Model file for the job. Use its own axes, mm. Round coordinates to 2 decimals unless told otherwise and drop trailing zeros. Loops run counter-clockwise (first coordinate to the right, second up) from the corner with the lowest first, then second, coordinate; pieces in that order, holes last. Notation, with made-up numbers: M -35.5,-27 L -19.5,-27 A19 ccw -19.5,-3 Z; hole C 62.5,32 d5. An arc over 180 degrees is marked long. Answer in a Markdown table with one row per item.
from build123d import *

# Parameters (mm, degrees)
SKETCH3_W                    = 720
SKETCH3_H                    = 30
BASE_FLANGE1_DEPTH           = 3
EDGE_FLANGE1_STRIP_W         = 13.4732
EDGE_FLANGE1_STRIP_H         = 3
EDGE_FLANGE1_STRIP_CUT_DEPTH = 720
EDGE_FLANGE1_DEPTH           = 720
SKETCH10_R                   = 5
CUT_EXTRUDE2_DEPTH           = 10
SKETCH11_R                   = 5
CUT_EXTRUDE3_DEPTH           = 10
SKETCH12_R                   = 5
CUT_EXTRUDE4_DEPTH           = 10


# Sheet-metal steps are written as plain solids
with BuildPart() as part:
    # Sketch3 → Base-Flange1 (new body)
    with BuildSketch(Plane(origin=(0, 0, 0), x_dir=(1, 0, 0), z_dir=(0, 1, 0))):
        Rectangle(SKETCH3_W, SKETCH3_H)
    extrude(amount=-BASE_FLANGE1_DEPTH)

    # Edge-Flange1 strip (across the edge) → Edge-Flange1 strip cut (cut)
    with BuildSketch(Plane(origin=(360, 0, -15), x_dir=(0, 0, 1), z_dir=(-1, 0, 0))):
        with Locations((-6, -1.5)):
            Rectangle(EDGE_FLANGE1_STRIP_W, EDGE_FLANGE1_STRIP_H)
    extrude(amount=EDGE_FLANGE1_STRIP_CUT_DEPTH, mode=Mode.SUBTRACT)

    # Edge-Flange1 section (across the edge) → Edge-Flange1 (add)
    with BuildSketch(Plane(origin=(360, 0, -15), x_dir=(0, 0, 1), z_dir=(-1, 0, 0))):
        with BuildLine():
            Line((-3, 0.7366), (-3, 27))
            Line((-3, 27), (0, 27))
            Line((0, 27), (0, 0.7366))
            ThreePointArc((0, 0.7366), (0.215745145, 0.215745145), (0.7366, 0))
            Line((0.7366, 0), (0.7366, -3))
            ThreePointArc((0.7366, -3), (-1.905575199, -1.905575199), (-3, 0.7366))
        make_face()
    extrude(amount=EDGE_FLANGE1_DEPTH)

    # Sketch10 → Cut-Extrude2 (cut)
    with BuildSketch(Plane(origin=(0, 0, 0), x_dir=(1, 0, 0), z_dir=(0, 1, 0))):
        with Locations(Location((-340, -1, 0), (0, 0, 270))):
            Circle(SKETCH10_R)
        with Locations(Location((-320, -1, 0), (0, 0, 270))):
            Circle(SKETCH10_R)
    cut_extrude2 = extrude(amount=-CUT_EXTRUDE2_DEPTH, mode=Mode.SUBTRACT)

    # Mirror1: Cut-Extrude2 across plane
    add(cut_extrude2.mirror(Plane(origin=(0, 0, 0), x_dir=(0, 0, 1), z_dir=(1, 0, 0))), mode=Mode.SUBTRACT)

    # Sketch11 → Cut-Extrude3 (cut)
    with BuildSketch(Plane.XY.offset(-15)):
        with Locations((225.5, 17)):
            Circle(SKETCH11_R)
        with Locations((-225.5, 17)):
            Circle(SKETCH11_R)
        with Locations((-150.5, 17)):
            Circle(SKETCH11_R)
        with Locations((150.5, 17)):
            Circle(SKETCH11_R)
        with Locations((50, 17)):
            Circle(SKETCH11_R)
        with Locations((-50, 17)):
            Circle(SKETCH11_R)
    extrude(amount=-CUT_EXTRUDE3_DEPTH, mode=Mode.SUBTRACT)

    # Sketch12 → Cut-Extrude4 (cut)
    with BuildSketch(Plane(origin=(0, 0, 0), x_dir=(1, 0, 0), z_dir=(0, 1, 0))):
        with Locations(Location((-75, -1, 0), (0, 0, 270))):
            Circle(SKETCH12_R)
        with Locations(Location((75, -1, 0), (0, 0, 270))):
            Circle(SKETCH12_R)
        with Locations(Location((135, -1, 0), (0, 0, 270))):
            Circle(SKETCH12_R)
        with Locations(Location((-135, -1, 0), (0, 0, 270))):
            Circle(SKETCH12_R)
    extrude(amount=-CUT_EXTRUDE4_DEPTH, mode=Mode.SUBTRACT)


solid = part.part
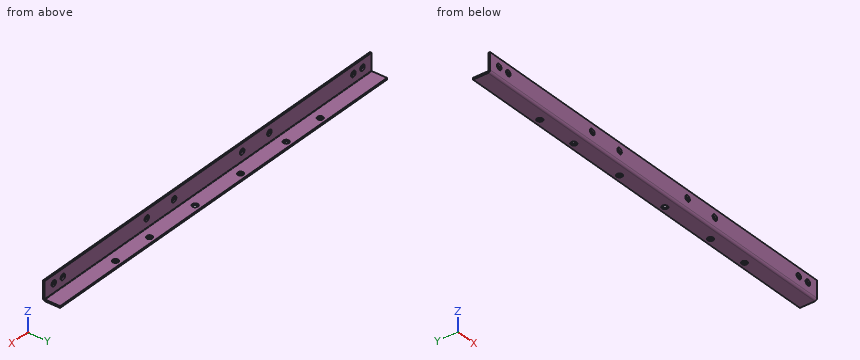
1. Wall check: probe 1 along Y at (x, z) = (-123, 9.5); probe 2 along Z at (x, y) = (-301.5, 18); probe 3 along Z at (x, y) = (73.5, -0.25). Give the ranges that are in metal, low to high.
Verdict:
| item | result |
|---|---|
| probe 1 | y = -3 to 0 |
| probe 2 | z = -18 to -15 |
| probe 3 | z = -17.87 to -3.77, 5.77 to 15 |
2. Pin check, flat tips, straight feed: pin 1 (1 mm diameter, centred on x = -176.5, y = 12.5, fed in from +Z); pin 2 (16 mm diameter, centred on x = 340, z = 1, fed in from +Y). Stop position of each tip, or through.
Verdict:
| item | result |
|---|---|
| pin 1 | stops at z = -15 |
| pin 2 | stops at y = 0 |
3. Saw through at A-A (y = 17). Write the cut outline in (x, z), and give its area (3 significant figures).
Verdict:
| item | result |
|---|---|
| outline | M -360,-18 L -230.5,-18 L -230.5,-15 L -360,-15 Z; M -220.5,-18 L -155.5,-18 L -155.5,-15 L -220.5,-15 Z; M -145.5,-18 L -55,-18 L -55,-15 L -145.5,-15 Z; M -45,-18 L 45,-18 L 45,-15 L -45,-15 Z; M 55,-18 L 145.5,-18 L 145.5,-15 L 55,-15 Z; M 155.5,-18 L 220.5,-18 L 220.5,-15 L 155.5,-15 Z; M 230.5,-18 L 360,-18 L 360,-15 L 230.5,-15 Z |
| area | 1,980 mm² |
4. Saw through at B-B (x = -281). Write the cut outline in (y, z), and give its area (3 significant figures).
Verdict:
| item | result |
|---|---|
| outline | M -3,-14.26 A3.74 ccw 0.74,-18 L 27,-18 L 27,-15 L 0.74,-15 A0.74 cw 0,-14.26 L 0,15 L -3,15 Z |
| area | 177 mm² |
5. Saw through at C-C (z = 1). State how many separate pieces and enclosed holes the cut face has, and give its area (3 significant figures).
Verdict:
| item | result |
|---|---|
| separate pieces | 9 |
| enclosed holes | 0 |
| area | 1,920 mm² |
